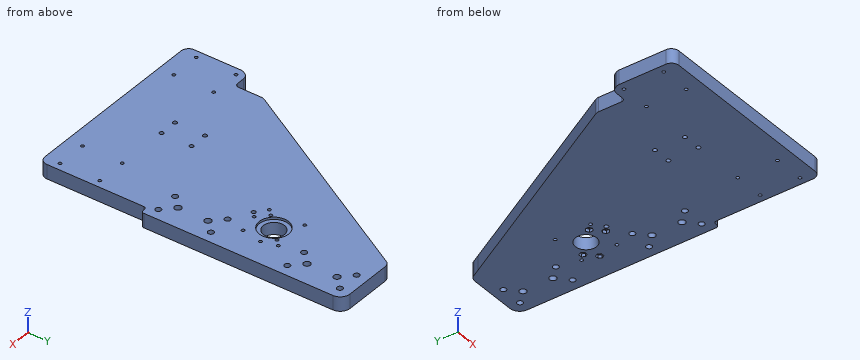
```python
from build123d import *

# Parameters (mm, degrees)
SKETCH2_W               = 270.829085825
SKETCH2_H               = 402
BOSS_EXTRUDE1_DEPTH     = 19
SKETCH3_W               = 7.829085824
SKETCH3_H               = 419.560715459
CUT_EXTRUDE1_DEPTH      = 20
CUT_EXTRUDE2_DEPTH      = 20
FILLET1_R               = 10
TAP_DRILL_FOR_M5_TAP1_D = 4.2
FILLET2_R               = 3
M7_CLEARANCE_HOLE1_D    = 7.6
SKETCH11_R              = 19.5
CUT_EXTRUDE4_DEPTH      = 32.266788686
CUT_EXTRUDE5_DEPTH      = 20
FILLET3_R               = 10
FILLET4_R               = 5
TAP_DRILL_FOR_M5_TAP2_D = 4.2
BOSS_EXTRUDE2_DEPTH     = 19
SKETCH16_R              = 19.5
SKETCH16_R_2            = 14
BOSS_EXTRUDE3_DEPTH     = 16
M5_CLEARANCE_HOLE4_D    = 5.5
M5_CLEARANCE_HOLE5_D    = 5.5
M8_CLEARANCE_HOLE1_D    = 9
TAP_DRILL_FOR_M5_TAP3_D = 4.2
CUT_EXTRUDE6_DEPTH      = 4


with BuildPart() as part:
    # Sketch2 → Boss-Extrude1 (new body)
    with BuildSketch(Plane.XY.offset(94)):
        with Locations((2322.392578952, 658.909518743)):
            Rectangle(SKETCH2_W, SKETCH2_H)
    extrude(amount=BOSS_EXTRUDE1_DEPTH)

    # Sketch3 → Cut-Extrude1 (cut)
    with BuildSketch(Plane.XY.offset(113)):
        with Locations((2190.892578951, 654.789569031)):
            Rectangle(SKETCH3_W, SKETCH3_H)
    extrude(amount=-CUT_EXTRUDE1_DEPTH, mode=Mode.SUBTRACT)

    # Sketch4 → Cut-Extrude2 (cut)
    with BuildSketch(Plane.XY.offset(113)):
        Polygon((2194.807121863, 532.656963015), (2380.609228318, 859.909518743), (2194.807121863, 859.909518743), align=None)
    extrude(amount=-CUT_EXTRUDE2_DEPTH, mode=Mode.SUBTRACT)

    # Fillet1
    fillet1_edges = [part.edges().sort_by_distance(p)[0] for p in [
        (2194.807121863, 457.909518743, 103.5),
        (2194.807121863, 532.656963015, 103.5),
        (2380.609228318, 859.909518743, 103.5),
        (2457.807121864, 457.909518743, 103.5),
    ]]
    fillet(fillet1_edges, radius=FILLET1_R)

    # Tap Drill for M5 Tap1 (through all)
    with Locations(Plane.XY.offset(113)):
        with Locations((2338.307121864, 531.660659234), (2314.307121864, 531.660659234), (2314.307121864, 571.660659234), (2338.307121864, 571.660659234), (2447.807121864, 531.160659234), (2447.807121864, 478.160659234), (2407.807121864, 478.160659234), (2407.807121864, 531.160659234), (2244.807121863, 531.160659234), (2244.807121863, 478.160659234), (2204.807121863, 478.160659234), (2204.807121863, 531.160659234)):
            Hole(TAP_DRILL_FOR_M5_TAP1_D / 2)

    # Fillet2
    fillet2_edges = [part.edges().sort_by_distance(p)[0] for p in [
        (2457.807121864, 859.909518743, 103.5),
    ]]
    fillet(fillet2_edges, radius=FILLET2_R)

    # M7 Clearance Hole1 (through all)
    with Locations(Plane.XY.offset(113)):
        with Locations((2422.807121864, 612.909518743), (2437.807121864, 627.909518743), (2452.807121864, 612.909518743), (2452.807121864, 682.909518743), (2437.807121864, 667.909518743), (2422.807121864, 682.909518743), (2452.807121864, 784.909518743), (2422.807121864, 854.909518743), (2452.807121864, 854.909518743), (2422.807121864, 784.909518743), (2437.807121864, 799.909518743), (2437.807121864, 839.909518743)):
            Hole(M7_CLEARANCE_HOLE1_D / 2)

    # Sketch11 → Cut-Extrude4 (cut)
    with BuildSketch(Plane.XY.offset(113)):
        with Locations((2405.807121866, 731.909518744)):
            Circle(SKETCH11_R)
    extrude(amount=-CUT_EXTRUDE4_DEPTH, mode=Mode.SUBTRACT)

    # Sketch12 → Cut-Extrude5 (cut)
    with BuildSketch(Plane.XY.offset(113)):
        Polygon((2221.807121863, 542.160659234), (2189.780449764, 542.160659234), (2221.807121863, 583.425794439), align=None)
    extrude(amount=-CUT_EXTRUDE5_DEPTH, mode=Mode.SUBTRACT)

    # Fillet3
    fillet3_edges = [part.edges().sort_by_distance(p)[0] for p in [
        (2200.202975144, 542.160659234, 103.5),
        (2221.807121863, 580.211962112, 103.5),
    ]]
    fillet(fillet3_edges, radius=FILLET3_R)

    # Fillet4
    fillet4_edges = [part.edges().sort_by_distance(p)[0] for p in [
        (2221.807121863, 542.160659234, 103.5),
    ]]
    fillet(fillet4_edges, radius=FILLET4_R)

    # Tap Drill for M5 Tap2 (through all)
    with Locations(Plane(origin=(0, 0, 94), x_dir=(-1, 0, 0), z_dir=(0, 0, -1))):
        with Locations((-2429.377121866, 755.479518745), (-2382.237121866, 755.479518745), (-2429.377121866, 708.339518745), (-2382.237121866, 708.339518745)):
            Hole(TAP_DRILL_FOR_M5_TAP2_D / 2)

    # Sketch15 → Boss-Extrude2 (add)
    with BuildSketch(Plane.XY.offset(113)):
        with BuildLine():
            Line((2457.807121864, 856.909518743), (2457.807121864, 597.10478226))
            ThreePointArc((2457.807121864, 597.10478226), (2458.978694739, 599.933209385), (2461.807121864, 601.10478226))
            Line((2461.807121864, 601.10478226), (2463.807121864, 601.10478226))
            ThreePointArc((2463.807121864, 601.10478226), (2466.635548988, 602.276355135), (2467.807121864, 605.10478226))
            Line((2467.807121864, 605.10478226), (2467.807121864, 856.909518743))
            ThreePointArc((2467.807121864, 856.909518743), (2463.999510019, 866.101906899), (2454.807121864, 869.909518743))
            Line((2454.807121864, 869.909518743), (2392.108600325, 869.909518743))
            ThreePointArc((2392.108600325, 869.909518743), (2387.077370287, 868.551666874), (2383.412473272, 864.846863605))
            Line((2383.412473272, 864.846863605), (2377.734836743, 854.846863605))
            ThreePointArc((2377.734836743, 854.846863605), (2381.399733758, 858.551666874), (2386.430963796, 859.909518743))
            Line((2386.430963796, 859.909518743), (2454.807121864, 859.909518743))
            ThreePointArc((2454.807121864, 859.909518743), (2456.928442207, 859.030839087), (2457.807121864, 856.909518743))
        make_face()
    extrude(amount=-BOSS_EXTRUDE2_DEPTH)

    # Sketch16 → Boss-Extrude3 (add)
    with BuildSketch(Plane(origin=(0, 0, 94), x_dir=(-1, 0, 0), z_dir=(0, 0, -1))):
        with Locations((-2405.807121866, 731.909518744)):
            Circle(SKETCH16_R)
        with Locations((-2405.807121866, 731.909518744)):
            Circle(SKETCH16_R_2, mode=Mode.SUBTRACT)
    extrude(amount=-BOSS_EXTRUDE3_DEPTH)

    # M5 Clearance Hole4 (through all)
    with Locations(Plane(origin=(0, 0, 94), x_dir=(-1, 0, 0), z_dir=(0, 0, -1))):
        with Locations((-2395.807121866, 697.409518744)):
            Hole(M5_CLEARANCE_HOLE4_D / 2)

    # M5 Clearance Hole5 (through all)
    with Locations(Plane(origin=(0, 0, 94), x_dir=(-1, 0, 0), z_dir=(0, 0, -1))):
        with Locations((-2338.307121864, 531.660659234), (-2314.307121864, 531.660659234), (-2314.307121864, 571.660659234), (-2338.307121864, 571.660659234)):
            Hole(M5_CLEARANCE_HOLE5_D / 2)

    # M8 Clearance Hole1 (through all)
    with Locations(Plane(origin=(0, 0, 94), x_dir=(-1, 0, 0), z_dir=(0, 0, -1))):
        with Locations((-2437.807121864, 627.909518743), (-2437.807121864, 667.909518743), (-2437.807121864, 799.909518743), (-2437.807121864, 839.909518743)):
            Hole(M8_CLEARANCE_HOLE1_D / 2)

    # Tap Drill for M5 Tap3 (through all)
    with Locations(Plane(origin=(0, 0, 94), x_dir=(-1, 0, 0), z_dir=(0, 0, -1))):
        with Locations((-2422.070577833, 748.172974712), (-2434.798499894, 735.445052651), (-2402.27158796, 702.918140716), (-2389.543665898, 715.646062777)):
            Hole(TAP_DRILL_FOR_M5_TAP3_D / 2)

    # Sketch25 → Cut-Extrude6 (cut)
    with BuildSketch(Plane(origin=(0, 0, 94), x_dir=(-1, 0, 0), z_dir=(0, 0, -1))):
        Polygon((-2430.208565254, 735.445052651), (-2432.503532574, 739.420052651), (-2437.093467214, 739.420052651), (-2439.388434534, 735.445052651), (-2437.093467214, 731.470052651), (-2432.503532574, 731.470052651), align=None)
        Polygon((-2426.660512473, 748.172974712), (-2424.365545153, 744.197974712), (-2419.775610513, 744.197974712), (-2417.480643193, 748.172974712), (-2419.775610513, 752.147974712), (-2424.365545153, 752.147974712), align=None)
        Polygon((-2402.27158796, 707.508075356), (-2406.24658796, 705.213108036), (-2406.24658796, 700.623173396), (-2402.27158796, 698.328206076), (-2398.29658796, 700.623173396), (-2398.29658796, 705.213108036), align=None)
        Polygon((-2389.543665898, 720.235997418), (-2393.518665898, 717.941030098), (-2393.518665898, 713.351095457), (-2389.543665898, 711.056128137), (-2385.568665898, 713.351095457), (-2385.568665898, 717.941030098), align=None)
    extrude(amount=-CUT_EXTRUDE6_DEPTH, mode=Mode.SUBTRACT)


solid = part.part
```
The model under review builds one solid part; all positions refer to its coordinate system, in mm. Give positions to 0.01 mm unless a question says otherwise; leave off trailing zeros. Write each loop counter-clockwise with the first axis right and the second up, starting at its lowest first coordinate (ties: lowest second). Pieces come first, ordered by that corner, then holes.
(1) Consider section A-A, the plane y = 726.5. Give the boundary of the cut face in (x, z).
(2) Consider section C-C, the plane y = 643. Give the boundary of the cut face in (x, z), and give its area (3 significant figures).
(3) To check wall thickness, follow L1, parallel to Y at x = 2453, z = 97.25; L2, parallel to Y at x = 2402, z = 105.75; L3, parallel to Y at x = 2425.5, z = 108.25. State the ranges of each line that lie inside material, in increasing order.
(4) Consider section D-D, the plane x = 2268. Give the boundary of the cut face in (y, z).
(5) For P1, Ø8, axis at y = 807, z = 99, coming from the -X side; P2, Ø1, axis at y = 673, z = 97, coming from the -X side; P3, Ø4, axis at x = 2436, y = 734.5, coming from the -Z side, all flat-tipped, find the tip position at first contact; note any pin that passes through.
(6) Consider section B-B, the plane z = 103.5. Give the number of separate pieces and of enclosed holes in the cut face, and give its area (3 significant figures).
Returned:
1. outline: (2304.86, 94) - (2392.89, 94) - (2392.89, 110) - (2387.07, 110) - (2387.07, 113) - (2304.86, 113) - close; (2418.72, 94) - (2467.81, 94) - (2467.81, 113) - (2424.54, 113) - (2424.54, 110) - (2418.72, 110) - close
2. outline: (2257.46, 94) - (2467.81, 94) - (2467.81, 113) - (2257.46, 113) - close
2. area: 4,000 mm2
3. L1: y = 459.36 to 609.11, 616.7 to 679.11, 686.7 to 781.11, 788.7 to 851.11, 858.7 to 869.91
3. L2: y = 457.91 to 700.84, 705 to 718.44, 745.38 to 869.91
3. L3: y = 457.91 to 610.23, 615.59 to 680.23, 685.59 to 782.23, 787.59 to 852.23, 857.59 to 869.91
4. outline: (457.91, 94) - (661.57, 94) - (661.57, 113) - (457.91, 113) - close
5. P1: stops at x = 2348.3
5. P2: stops at x = 2274.2
5. P3: stops at z = 98
6. separate pieces: 1
6. enclosed holes: 34
6. area: 76,700 mm2
